Could you check a few things on this model? Use its own coordinates, in mm. Face numbers are marked on the shaded views. A direction names the side the tool comes from. Round coordinates to 2 decimals unless told otherwise and drop trailing zeros. Loops run counter-clockwise (first coordinate to the right, second up) from the corner with the lowest first, then second, coordinate; pieces in that order, holes last. Notation, with made-up numbers: (52.25, 34.25) -> (109.25, 34.25) arc R17 ccw to (109.25, 41.25) -> close; hole circle Ø10 at (-9, 46). An arc over 180 degrees is marked (long way). One line per item, written item: value.
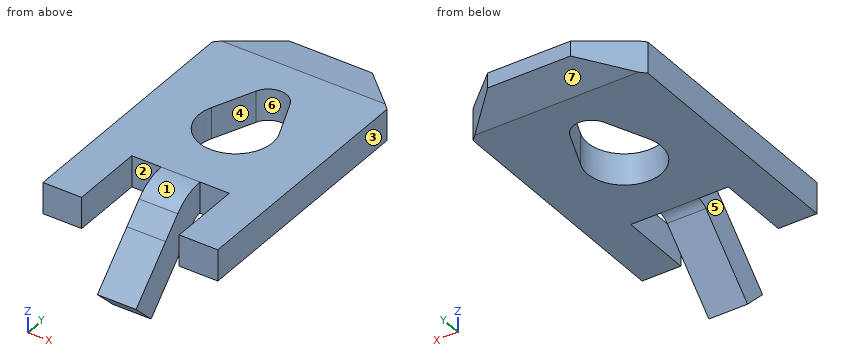
```python
from build123d import *

# Parameters (mm, degrees)
BOSS_EXTRUDE1_DEPTH    = 4.75
CUT_EXTRUDE1_REACH     = 11.471
CUT_EXTRUDE2_DEPTH     = 0.85
SKETCH6_W              = 0.8
SKETCH6_H              = 2
CUT_EXTRUDE3_DEPTH     = 0.85
SKETCH7_W              = 1.05
SKETCH7_H              = 0.85
BOSS_EXTRUDE2_DEPTH    = 1
SKETCHED_START         = 1.85
SKETCHED_BEND1_DEPTH   = 1.05
SKETCHED_BEND1_2_DEPTH = 1.05


# Read off the part's stored shape, not the designer's step: Sketched Bend1
with BuildPart() as part:
    # Sketch1 → Boss-Extrude1 (new body)
    with BuildSketch(Plane(origin=(0, 0, 0), x_dir=(0, 0, -1), z_dir=(1, 0, 0))):
        Polygon((0, 0.15), (0, 7.05), (-0.241393443, 8.15), (-0.647131148, 8.15), (-0.85, 7.05), (-0.85, 0.15), align=None)
    extrude(amount=BOSS_EXTRUDE1_DEPTH)

    # Cut-Extrude1: up to this face of the body (flat: up to its plane)
    cut_extrude1_end = Plane(part.part.faces().sort_by_distance((2.375, 3.6, 0))[0])
    # Sketch4 → Cut-Extrude1 (cut, up to the picked face)
    with BuildSketch(Plane.XY.offset(0.85), mode=Mode.PRIVATE) as cut_extrude1_sk1:
        Polygon((0, 6.9), (1.25, 8.15), (0, 8.15), align=None)
    cut_extrude1_tool1 = split(extrude(cut_extrude1_sk1.sketch, amount=-CUT_EXTRUDE1_REACH, mode=Mode.PRIVATE), bisect_by=cut_extrude1_end, keep=Keep.BOTH, mode=Mode.PRIVATE)
    # Sketch4 → Cut-Extrude1 (cut, up to the picked face)
    with BuildSketch(Plane.XY.offset(0.85), mode=Mode.PRIVATE) as cut_extrude1_sk2:
        Polygon((3.5, 8.15), (4.75, 6.9), (4.75, 8.15), align=None)
    cut_extrude1_tool2 = split(extrude(cut_extrude1_sk2.sketch, amount=-CUT_EXTRUDE1_REACH, mode=Mode.PRIVATE), bisect_by=cut_extrude1_end, keep=Keep.BOTH, mode=Mode.PRIVATE)
    add(cut_extrude1_tool1.solids().sort_by(Axis((0.416667, 7.733333, 0.85), (0, 0, -1)))[0], mode=Mode.SUBTRACT)
    add(cut_extrude1_tool2.solids().sort_by(Axis((4.333333, 7.733333, 0.85), (0, 0, -1)))[0], mode=Mode.SUBTRACT)

    # Sketch5 → Cut-Extrude2 (cut)
    with BuildSketch(Plane.XY.offset(0.85)):
        with BuildLine():
            Line((1.913461538, 5.842307692), (1.451923077, 4.734615385))
            ThreePointArc((1.451923077, 4.734615385), (2.37510742, 3.350000006), (3.297994271, 4.734813689))
            Line((3.297994271, 4.734813689), (2.842436975, 5.827489929))
            ThreePointArc((2.842436975, 5.827489929), (2.382974312, 6.149936406), (1.913461538, 5.842307692))
        make_face()
    extrude(amount=-CUT_EXTRUDE2_DEPTH, mode=Mode.SUBTRACT)

    # Sketch6 → Cut-Extrude3 (cut)
    with BuildSketch(Plane(origin=(0, 0, 0), x_dir=(-1, 0, 0), z_dir=(0, 0, -1))):
        with Locations((-3.3, 1.15)):
            Rectangle(SKETCH6_W, SKETCH6_H)
        with Locations((-1.45, 1.15)):
            Rectangle(SKETCH6_W, SKETCH6_H)
    extrude(amount=-CUT_EXTRUDE3_DEPTH, mode=Mode.SUBTRACT)

    # Sketch7 → Boss-Extrude2 (add)
    with BuildSketch(Plane.XZ.offset(-0.15)):
        with Locations((2.375, 0.425)):
            Rectangle(SKETCH7_W, SKETCH7_H)
    extrude(amount=BOSS_EXTRUDE2_DEPTH)

    # Sketched Bend1 outline → Sketched Bend1 (cut)
    with BuildSketch(Plane.YZ.offset(SKETCHED_START)):
        with BuildLine():
            ThreePointArc((1.266116524, 0.483883476), (1.67164571, 0.754849416), (2.15, 0.85))
            Line((2.15, 0.85), (-0.85, 0.85))
            Line((-0.85, 0.85), (-0.85, 0))
            Line((-0.85, 0), (0.782233048, 0))
            Line((0.782233048, 0), (1.266116524, 0.483883476))
        make_face()
    extrude(amount=SKETCHED_BEND1_DEPTH, mode=Mode.SUBTRACT)

    # Sketched Bend1 2 outline → Sketched Bend1 2 (add)
    with BuildSketch(Plane.YZ.offset(SKETCHED_START)):
        with BuildLine():
            Line((2.15, 0), (0.782233048, 0))
            Line((0.782233048, 0), (-0.397031517, -1.179264564))
            Line((-0.397031517, -1.179264564), (0.204009247, -1.780305328))
            Line((0.204009247, -1.780305328), (1.867157288, -0.117157288))
            ThreePointArc((1.867157288, -0.117157288), (1.996926627, -0.030448187), (2.15, 0))
        make_face()
    extrude(amount=SKETCHED_BEND1_2_DEPTH)


solid = part.part
```
(1) Imagine slicing it at C-C on y = 0.5. Write out the boundary of the cut face in (x, z).
Results below:
outline: (0, 0) -> (1.05, 0) -> (1.05, 0.85) -> (0, 0.85) -> close; (1.85, -1.48) -> (2.9, -1.48) -> (2.9, -0.28) -> (1.85, -0.28) -> close; (3.7, 0) -> (4.75, 0) -> (4.75, 0.85) -> (3.7, 0.85) -> close
(2) For pin 1 Ø0.9 at (x, z) = (4.5, 0.5) entering from -Y; pin 2 Ø1.5 at (x, z) = (2, 0) entering from -Y; pin 3 Ø1.2 at (x, y) = (2.375, 4.35) entering from -Z, each with a flat end and sliding along its axis, tell me the tip position at first contact or that it passes through.
Results below:
pin 1: stops at y = 0.15
pin 2: stops at y = 0.03
pin 3: passes through
(3) We'd pull the mould along Y, two halves only. Please class the marked faces 5, 6 and 7: +Y half, -Y half, draft (parallel to the pull), parting line (faces both ways), or undercut.
Results below:
face 5: draft
face 6: undercut
face 7: +Y half
(4) Imagine slicing it at B-B on x = 1.7. Write out the boundary of the cut face in (y, z).
Results below:
outline: (2.15, 0) -> (3.61, 0) -> (3.61, 0.85) -> (2.15, 0.85) -> close; (5.33, 0) -> (7.05, 0) -> (8.15, 0.24) -> (8.15, 0.65) -> (7.05, 0.85) -> (5.33, 0.85) -> close
(5) Imagine slicing it at D-D on z = 0.1. Write out the boundary of the cut face in (x, y) (3 decimals).
Results below:
outline: (0, 0.15) -> (1.05, 0.15) -> (1.05, 2.15) -> (1.85, 2.15) -> (1.85, 0.882) -> (2.9, 0.882) -> (2.9, 2.15) -> (3.7, 2.15) -> (3.7, 0.15) -> (4.75, 0.15) -> (4.75, 6.9) -> (4.144, 7.506) -> (0.606, 7.506) -> (0, 6.9) -> close; hole (1.452, 4.735) arc R1 ccw (long way) to (3.298, 4.735) -> (2.842, 5.827) arc R0.5 ccw to (1.913, 5.842) -> close
(6) Imagine slicing it at A-A on y = 4.35. Write out the boundary of the cut face in (x, z) (3 decimals), then the cut area to 3 significant figures.
Results below:
outline: (0, 0) -> (1.375, 0) -> (1.375, 0.85) -> (0, 0.85) -> close; (3.375, 0) -> (4.75, 0) -> (4.75, 0.85) -> (3.375, 0.85) -> close
area: 2.34 mm²
(7) Please list where these lines run through material, in increasing order: L1, parallel to X at y = 4.35, z = 0.3 (3 decimals); L2, parallel to Z at x = 1.45, y = 5.5; L3, parallel to X at y = 0.5, z = -0.7.
Results below:
L1: x = 0 to 1.375, 3.375 to 4.75
L2: z = 0 to 0.85
L3: x = 1.85 to 2.9
(8) On a 3-axis mill with a long thin cutter (end or side, diameter ignored), from which of +Z, -Z, +X, -X, +Y, -Y can I reach the whole of each face in a straight line? I mean the marked faces 1, 2, 3 and 4. Say none if no direction works.
Results below:
face 1: +Z, -Y
face 2: +Z, -Z, -Y
face 3: +Z, -Z, +X, +Y, -Y
face 4: +Z, -Z
